Autodesk Fusion 360 part; units mm, degrees
sketch "Sketch1" plane through (0, 0, 0) normal (0, 0, 1) x (1, 0, 0)
  line L0 (-21.15, 21.15) -> (21.15, 21.15)
  line L1 (21.15, 21.15) -> (21.15, -21.15)
  line L2 (21.15, -21.15) -> (-21.15, -21.15)
  line L3 (-21.15, -21.15) -> (-21.15, 21.15)
  line L4 (-21.15, 21.15) -> (21.15, -21.15) construction
  line L5 (21.15, 21.15) -> (-21.15, -21.15) construction
  line L6 (-15.5, 15.5) -> (15.5, 15.5) construction
  line L7 (15.5, 15.5) -> (15.5, -15.5) construction
  line L8 (15.5, -15.5) -> (-15.5, -15.5) construction
  line L9 (-15.5, -15.5) -> (-15.5, 15.5) construction
  line L10 (-15.5, 15.5) -> (15.5, -15.5) construction
  line L11 (15.5, 15.5) -> (-15.5, -15.5) construction
  circle A0 centre (-15.5, 15.5) radius 1.5
  circle A1 centre (-15.5, -15.5) radius 1.5
  circle A2 centre (15.5, -15.5) radius 1.5
  circle A3 centre (15.5, 15.5) radius 1.5
  circle A4 centre (0, 0) radius 2.5
  circle A5 centre (0, 0) radius 11
  line L12 (-21.15, -21.15) -> (-24.15, -21.15)
  line L13 (-24.15, -21.15) -> (-24.15, 21.15)
  line L14 (-24.15, 21.15) -> (-21.15, 21.15)
  line L15 (-21.15, 21.15) -> (-21.15, -21.15)
  line L16 (21.15, -21.15) -> (24.15, -21.15)
  line L17 (24.15, -21.15) -> (24.15, 21.15)
  line L18 (24.15, 21.15) -> (21.15, 21.15)
  line L19 (21.15, 21.15) -> (21.15, -21.15)
  dimension "d1" = 42.3
  dimension "d2" = 42.3
  dimension "d5" = 31
  dimension "d6" = 31
  dimension "d8" = 3
  dimension "d10" = 360
  dimension "d12" = 5
  dimension "d14" = 22
  dimension "d17" = 3
  dimension "d18" = 42.3
  dimension "d19" = 3
  dimension "d20" = 42.3
extrude "Extrude1" add sketch "Sketch1" along normal blind 5 contours L0 L1 L2 L3 L15 L19 | L3 L12 L13 L14 L15 | L1 L16 L17 L18 L19 | A5
extrude "Extrude2" add sketch "Sketch1" against normal blind 24 contours L3 L12 L13 L14 L15 | L1 L16 L17 L18 L19
extrude "Extrude3" cut sketch "Sketch1" along normal blind 2 contours A5
sketch "Sketch2" plane through (24.15, 0, 0) normal (1, 0, 0) x (0, 1, 0)
  line L0 (-21.15, 5) -> (-21.15, -24)
  line L1 (-21.15, -24) -> (21.15, -24)
  line L2 (21.15, -24) -> (21.15, 5)
  line L3 (-21.15, -24) -> (21.15, -24)
  line L4 (21.15, -24) -> (21.15, -21)
  line L5 (21.15, -21) -> (-21.15, -21)
  line L6 (-21.15, -21) -> (-21.15, -24)
  line L7 (21.15, 5) -> (-21.15, 5)
  dimension "d28" = 42.3
  dimension "d29" = 3
extrude "Extrude4" add sketch "Sketch2" along normal blind 10 contours L0 L1 L2 L3 L4 L5 L6
sketch "Sketch3" plane through (-24.15, 0, 0) normal (-1, 0, 0) x (0, -1, 0)
  line L0 (21.15, -24) -> (21.15, 5)
  line L1 (21.15, 5) -> (-21.15, 5)
  line L2 (-21.15, 5) -> (-21.15, -24)
  line L3 (-21.15, -24) -> (21.15, -24)
  line L4 (-21.15, -24) -> (21.15, -24)
  line L5 (21.15, -24) -> (21.15, -21)
  line L6 (21.15, -21) -> (-21.15, -21)
  line L7 (-21.15, -21) -> (-21.15, -24)
  dimension "d32" = 42.3
  dimension "d33" = 3
extrude "Extrude5" add sketch "Sketch3" along normal blind 10 contours L0 L2 L3 L4 L5 L6 L7
sketch "Sketch4" plane through (0, 0, -21) normal (0, 0, 1) x (-1, 0, 0)
  line L0 (24.15, 21.15) -> (24.15, -21.15)
  line L1 (24.15, -21.15) -> (34.15, -21.15)
  line L2 (34.15, -21.15) -> (34.15, 21.15)
  line L3 (34.15, 21.15) -> (24.15, 21.15)
  line L4 (24.15, 0) -> (34.15, 0) construction
  line L5 (29.15, 0) -> (29.15, 10) construction
  circle A0 centre (29.15, 10) radius 2.5
  circle A1 centre (29.15, -10) radius 2.5
  dimension "d36" = 10
  dimension "d38" = 5
extrude "Extrude6" cut sketch "Sketch4" against normal blind 3 contours A0 | A1
sketch "Sketch5" plane through (0, 0, -21) normal (0, 0, 1) x (-1, 0, 0)
  line L0 (-24.15, -21.15) -> (-24.15, 21.15)
  line L1 (-24.15, 21.15) -> (-34.15, 21.15)
  line L2 (-34.15, 21.15) -> (-34.15, -21.15)
  line L3 (-34.15, -21.15) -> (-24.15, -21.15)
  line L4 (-34.15, 0) -> (-24.15, 0) construction
  line L5 (-29.15, 0) -> (-29.15, 10) construction
  circle A0 centre (-29.15, 10) radius 2.5
  circle A1 centre (-29.15, -10) radius 2.5
  dimension "d41" = 10
  dimension "d42" = 5
extrude "Extrude7" cut sketch "Sketch5" against normal blind 3 contours A0 | A1
fillet "Fillet1" radius 3 4 edges at (34.15, 21.15, -22.5) (34.15, -21.15, -22.5) (-34.15, 21.15, -22.5) (-34.15, -21.15, -22.5)
fillet "Fillet2" radius 4 2 edges at (24.15, 0, 5) (-24.15, 0, 5)
fillet "Fillet3" radius 1 2 edges at (21.15, 0, 0) (-21.15, 0, 0)
fillet "Fillet3" radius 1 2 edges at (24.15, 0, -21) (-24.15, 0, -21)
equation "d1 = nema_l"
equation "d2 = nema_l"
equation "nema_l = 42.3 mm"
equation "nema_spacing = 31 mm"
equation "d5 = nema_spacing"
equation "d6 = nema_spacing"
equation "nema_hole = 3 mm"
equation "d8 = nema_hole"
equation "nema_shaft = 5 mm"
equation "d12 = nema_shaft"
equation "nema_disc = 22 mm"
equation "d14 = nema_disc"
equation "thick_vert = 3 mm"
equation "thick_hori = 3 mm"
equation "d17 = thick_vert"
equation "d18 = nema_l"
equation "d19 = thick_vert"
equation "d20 = nema_l"
equation "d21 = 2 mm + thick_hori"
equation "height = 24 mm"
equation "d28 = nema_l"
equation "d29 = thick_hori"
equation "d32 = nema_l"
equation "d33 = thick_hori"
equation "alu_hole = 5 mm"
equation "d38 = alu_hole"
equation "d42 = alu_hole"
Could you check a few things on this model? Use its own coordinates, in mm. A direction names the side the tool comes from. Coordinates: 2 decimals unless noted, no trailing zeros. Loops run counter-clockwise (first coordinate to the right, second up) from the corner with the lowest first, then second, coordinate; pieces in that order, holes last. Notation, with made-up numbers: M 69,32 L 91,32 A17 ccw 91,47 Z; hole C 55,12.5 d9. An arc over 180 degrees is marked long. Put each result on its own line as item: value. Start each with the question number.
(1) I need wall thicknesses on line 1 (Y direction, x = -15.5, z = 3.9); line 2 (X direction, y = -10, z = -22.75); line 3 (X direction, y = -10, z = -4.5). Which ranges of each line are inside material? Lowest first, please. Write a range as from..to.
(2) Suppose I cut it at B-B on y = -15.5. Please give me the cut outline in (x, z).
(3) Suppose I cut it at C-C on z = -9. Please give me the cut outline in (x, y), then the cut area to 3 significant figures.
(4) Will these pins go through, and if not, where does the flat tip stop? P1, Ø11.5, axis at y = -3, z = -11, coming from the +X side; P2, Ø20, axis at x = -1.5, y = 8, coming from the -Z side; P3, Ø8, axis at y = -0.5, z = -10.5, coming from the -X side.
(5) Suppose I cut it at A-A on x = -15.5. Please give me the cut outline in (y, z).
(6) Thinking about a two-plate mould opening in Y: for faces 5 (the face through (-33.29, -20.25, -22.48)), 6 (the face through (0.1, 21.15, 0.2)), 7 (the face through (14, -15.57, 2.46)), 8 (the face through (24.15, 0, -10)), which applies, pulls with the +Y half, pulls with the -Y half, needs draft (parallel to the pull), parting line crosses it, or undercut?
(7) Suppose I cut it at D-D on x = 0. Please give me the cut outline in (y, z).
(8) For faces 1 (the face through (-2.38, 10.74, 0.99)), 2 (the face through (-24.15, 0, -10)), 3 (the face through (9, 10, 0)), 4 (the face through (-33.29, 20.25, -22.52)), which set-ups out of +Z, -Z, +X, -X, +Y, -Y let a thin tool reach every point of the face, with its end or its side?
Solutions:
1. line 1: y = -21.15..-17, -14..14, 17..21.15
1. line 2: x = -34.15..-31.65, -26.65..-21.15, 21.15..26.65, 31.65..34.15
1. line 3: x = -24.15..-21.15, 21.15..24.15
2. outline: M -34.15,-24 L -21.15,-24 L -21.15,-1 A1 cw -20.15,0 L -17,0 L -17,5 L -20.15,5 A4 ccw -24.15,1 L -24.15,-20 A1 cw -25.15,-21 L -34.15,-21 Z; M -14,0 L 14,0 L 14,5 L -14,5 Z; M 17,0 L 20.15,0 A1 cw 21.15,-1 L 21.15,-24 L 34.15,-24 L 34.15,-21 L 25.15,-21 A1 cw 24.15,-20 L 24.15,1 A4 ccw 20.15,5 L 17,5 Z
3. outline: M -24.15,-21.15 L -21.15,-21.15 L -21.15,21.15 L -24.15,21.15 Z; M 21.15,-21.15 L 24.15,-21.15 L 24.15,21.15 L 21.15,21.15 Z
3. area: 254 mm2
4. P1: stops at x = 24.15
4. P2: stops at z = 0
4. P3: stops at x = -24.15
5. outline: M -21.15,0 L -17,0 L -17,5 L -21.15,5 Z; M -14,0 L 14,0 L 14,5 L -14,5 Z; M 17,0 L 21.15,0 L 21.15,5 L 17,5 Z
6. face 5: pulls with the -Y half
6. face 6: pulls with the +Y half
6. face 7: undercut
6. face 8: needs draft
7. outline: M -21.15,0 L -11,0 L -11,2 L -2.5,2 L -2.5,5 L -21.15,5 Z; M 2.5,2 L 11,2 L 11,0 L 21.15,0 L 21.15,5 L 2.5,5 Z
8. face 1: -Z
8. face 2: +Z, -X, +Y, -Y
8. face 3: -Z, +Y, -Y
8. face 4: +Z, -Z, -X, +Y
